from build123d import *

# Parameters (mm, degrees)
F0_R     = 20
F0_R_2   = 3
F1_DEPTH = 15
F2_R     = 1.5
F3_DEPTH = 15
F4_COUNT = 30


with BuildPart() as f1:
    # F0 (on Front) → F1 (new body)
    with BuildSketch(Plane.XZ):
        Circle(F0_R)
        Circle(F0_R_2, mode=Mode.SUBTRACT)
    extrude(amount=F1_DEPTH)


with BuildPart() as f3:
    # F2 (on face) → F3 (new body, through all)
    with BuildSketch(Plane.XZ.offset(15)):
        with Locations((20.171481, 1.781533)):
            Circle(F2_R)
    extrude(amount=-F3_DEPTH)


with BuildPart() as f4_1:
    # F4: instance of F3
    add(f3.part.rotate(Axis((0, 0, 0), (0, 1, 0)), 1 * 360 / F4_COUNT))


with BuildPart() as f4_2:
    # F4: instance of F3
    add(f3.part.rotate(Axis((0, 0, 0), (0, 1, 0)), 2 * 360 / F4_COUNT))


with BuildPart() as f4_3:
    # F4: instance of F3
    add(f3.part.rotate(Axis((0, 0, 0), (0, 1, 0)), 3 * 360 / F4_COUNT))


with BuildPart() as f4_4:
    # F4: instance of F3
    add(f3.part.rotate(Axis((0, 0, 0), (0, 1, 0)), 4 * 360 / F4_COUNT))


with BuildPart() as f4_5:
    # F4: instance of F3
    add(f3.part.rotate(Axis((0, 0, 0), (0, 1, 0)), 5 * 360 / F4_COUNT))


with BuildPart() as f4_6:
    # F4: instance of F3
    add(f3.part.rotate(Axis((0, 0, 0), (0, 1, 0)), 6 * 360 / F4_COUNT))


with BuildPart() as f4_7:
    # F4: instance of F3
    add(f3.part.rotate(Axis((0, 0, 0), (0, 1, 0)), 7 * 360 / F4_COUNT))


with BuildPart() as f4_8:
    # F4: instance of F3
    add(f3.part.rotate(Axis((0, 0, 0), (0, 1, 0)), 8 * 360 / F4_COUNT))


with BuildPart() as f4_9:
    # F4: instance of F3
    add(f3.part.rotate(Axis((0, 0, 0), (0, 1, 0)), 9 * 360 / F4_COUNT))


with BuildPart() as f4_10:
    # F4: instance of F3
    add(f3.part.rotate(Axis((0, 0, 0), (0, 1, 0)), 10 * 360 / F4_COUNT))


with BuildPart() as f4_11:
    # F4: instance of F3
    add(f3.part.rotate(Axis((0, 0, 0), (0, 1, 0)), 11 * 360 / F4_COUNT))


with BuildPart() as f4_12:
    # F4: instance of F3
    add(f3.part.rotate(Axis((0, 0, 0), (0, 1, 0)), 12 * 360 / F4_COUNT))


with BuildPart() as f4_13:
    # F4: instance of F3
    add(f3.part.rotate(Axis((0, 0, 0), (0, 1, 0)), 13 * 360 / F4_COUNT))


with BuildPart() as f4_14:
    # F4: instance of F3
    add(f3.part.rotate(Axis((0, 0, 0), (0, 1, 0)), 14 * 360 / F4_COUNT))


with BuildPart() as f4_15:
    # F4: instance of F3
    add(f3.part.rotate(Axis((0, 0, 0), (0, 1, 0)), 15 * 360 / F4_COUNT))


with BuildPart() as f4_16:
    # F4: instance of F3
    add(f3.part.rotate(Axis((0, 0, 0), (0, 1, 0)), 16 * 360 / F4_COUNT))


with BuildPart() as f4_17:
    # F4: instance of F3
    add(f3.part.rotate(Axis((0, 0, 0), (0, 1, 0)), 17 * 360 / F4_COUNT))


with BuildPart() as f4_18:
    # F4: instance of F3
    add(f3.part.rotate(Axis((0, 0, 0), (0, 1, 0)), 18 * 360 / F4_COUNT))


with BuildPart() as f4_19:
    # F4: instance of F3
    add(f3.part.rotate(Axis((0, 0, 0), (0, 1, 0)), 19 * 360 / F4_COUNT))


with BuildPart() as f4_20:
    # F4: instance of F3
    add(f3.part.rotate(Axis((0, 0, 0), (0, 1, 0)), 20 * 360 / F4_COUNT))


with BuildPart() as f4_21:
    # F4: instance of F3
    add(f3.part.rotate(Axis((0, 0, 0), (0, 1, 0)), 21 * 360 / F4_COUNT))


with BuildPart() as f4_22:
    # F4: instance of F3
    add(f3.part.rotate(Axis((0, 0, 0), (0, 1, 0)), 22 * 360 / F4_COUNT))


with BuildPart() as f4_23:
    # F4: instance of F3
    add(f3.part.rotate(Axis((0, 0, 0), (0, 1, 0)), 23 * 360 / F4_COUNT))


with BuildPart() as f4_24:
    # F4: instance of F3
    add(f3.part.rotate(Axis((0, 0, 0), (0, 1, 0)), 24 * 360 / F4_COUNT))


with BuildPart() as f4_25:
    # F4: instance of F3
    add(f3.part.rotate(Axis((0, 0, 0), (0, 1, 0)), 25 * 360 / F4_COUNT))


with BuildPart() as f4_26:
    # F4: instance of F3
    add(f3.part.rotate(Axis((0, 0, 0), (0, 1, 0)), 26 * 360 / F4_COUNT))


with BuildPart() as f4_27:
    # F4: instance of F3
    add(f3.part.rotate(Axis((0, 0, 0), (0, 1, 0)), 27 * 360 / F4_COUNT))


with BuildPart() as f4_28:
    # F4: instance of F3
    add(f3.part.rotate(Axis((0, 0, 0), (0, 1, 0)), 28 * 360 / F4_COUNT))


with BuildPart() as f4_29:
    # F4: instance of F3
    add(f3.part.rotate(Axis((0, 0, 0), (0, 1, 0)), 29 * 360 / F4_COUNT))


with BuildPart() as f1_1:
    add(f1.part)

    # F5: cut F4_15, F4_16, F4_17, F4_18, F4_19, F4_20, F4_21, F4_23, F4_25, F4_22, F4_24, F4_26, F4_27, F4_28, F4_29, F3, F4_1, F4_2, F4_3, F4_4, F4_5, F4_6, F4_7, F4_8, F4_9, F4_10, F4_11, F4_12, F4_13, F4_14
    add(f4_15.part, mode=Mode.SUBTRACT)
    add(f4_16.part, mode=Mode.SUBTRACT)
    add(f4_17.part, mode=Mode.SUBTRACT)
    add(f4_18.part, mode=Mode.SUBTRACT)
    add(f4_19.part, mode=Mode.SUBTRACT)
    add(f4_20.part, mode=Mode.SUBTRACT)
    add(f4_21.part, mode=Mode.SUBTRACT)
    add(f4_23.part, mode=Mode.SUBTRACT)
    add(f4_25.part, mode=Mode.SUBTRACT)
    add(f4_22.part, mode=Mode.SUBTRACT)
    add(f4_24.part, mode=Mode.SUBTRACT)
    add(f4_26.part, mode=Mode.SUBTRACT)
    add(f4_27.part, mode=Mode.SUBTRACT)
    add(f4_28.part, mode=Mode.SUBTRACT)
    add(f4_29.part, mode=Mode.SUBTRACT)
    add(f3.part, mode=Mode.SUBTRACT)
    add(f4_1.part, mode=Mode.SUBTRACT)
    add(f4_2.part, mode=Mode.SUBTRACT)
    add(f4_3.part, mode=Mode.SUBTRACT)
    add(f4_4.part, mode=Mode.SUBTRACT)
    add(f4_5.part, mode=Mode.SUBTRACT)
    add(f4_6.part, mode=Mode.SUBTRACT)
    add(f4_7.part, mode=Mode.SUBTRACT)
    add(f4_8.part, mode=Mode.SUBTRACT)
    add(f4_9.part, mode=Mode.SUBTRACT)
    add(f4_10.part, mode=Mode.SUBTRACT)
    add(f4_11.part, mode=Mode.SUBTRACT)
    add(f4_12.part, mode=Mode.SUBTRACT)
    add(f4_13.part, mode=Mode.SUBTRACT)
    add(f4_14.part, mode=Mode.SUBTRACT)

    # F6 (on Right) → F7 (revolve)
    with BuildSketch(Plane.YZ):
        Polygon((-15, 3), (-15, 0), (90, 0), (90, 16), (40, 16), (40, 15), (10, 15), (10, 3), align=None)
    revolve(axis=Axis((0, 37.5, 0), (0, 1, 0)))


solid = f1_1.part
Part model, mm, in its own coordinate system. A direction names the side the tool comes from. Coordinates: 2 decimals unless noted, no trailing zeros. Order: outer loops, then holes, each group sorted by start corner. A loop starts at its lowest first (then second) coordinate and runs counter-clockwise, first axis right, second up. Notation, with made-up numbers: M -17,13.5 L -10,13.5 A24 cw -10,29.5 Z; hole C 13,-38 d5. An arc over 180 degrees is marked long. Use a Markdown table: item, result.
(1) Probe L1, parallel to Y at x = 11, z = -4; L2, parallel to Y at x = 18.5, z = -4; L3, parallel to X at y = 2, z = 0. List the from-to ranges inside material, lowest first.
A:
| item | result |
|---|---|
| L1 | y = -15 to 0, 10 to 90 |
| L2 | y = -15 to 0 |
| L3 | x = -3 to 3 |
(2) Cut at B-B on y = 3. Write the cut outline in (x, z).
A:
| item | result |
|---|---|
| outline | C 0,0 d6 |
(3) Tool access for faces 1 (the cylindrical face through (-10.791, -7.605, 15.334)), 2 (the cylindrical face through (0.9, 4.93, 2.86)): list every direction of +Z, -Z, +X, -X, +Y, -Y with a clear straight run to the whole face (end or side of a thin tool).
A:
| item | result |
|---|---|
| face 1 | +Y, -Y |
| face 2 | none |
(4) Pull direction Z, two halves, no side cores. Call faces 3 (the flat face through (0, -15, 0)), 4 (the cylindrical face through (13.7, -7.6, -12.8)), 5 (the cylindrical face through (3.6, -7.6, -18.4)), 6 (the cylindrical face through (16.378, -7.605, 9.129)): released by +Z, released by -Z, zero draft, split by the parting line, or undercut.
A:
| item | result |
|---|---|
| face 3 | zero draft |
| face 4 | undercut |
| face 5 | released by -Z |
| face 6 | undercut |
(5) Cut at A-A on x = 0. Write the cut outline in (y, z), then the cut area to 3 significant figures.
A:
| item | result |
|---|---|
| outline | M -15,-18.79 L 0,-18.79 L 0,-3 L 10,-3 L 10,-15 L 40,-15 L 40,-16 L 90,-16 L 90,16 L 40,16 L 40,15 L 10,15 L 10,3 L 0,3 L 0,18.79 L -15,18.79 Z |
| area | 3,120 mm^2 |
(6) Cut at C-C on y = 35.5. Write the cut outline in (x, z).
A:
| item | result |
|---|---|
| outline | C 0,0 d30 |
(7) Flat gauge pins, fed straight in: pin 1 (12 mm diameter, centred on x = -15, z = 15, fed in from +Y); pin 2 (5 mm diameter, centred on x = 3.5, y = 56.5, fed in from +Z); pin 3 (1 mm diameter, centred on y = 46, z = -2.5, fed in from +X); pin 4 (2 mm diameter, centred on x = 6, y = -1.5, fed in from +Z). Where does each tip first touch, or does it go through?
A:
| item | result |
|---|---|
| pin 1 | stops at y = 90 |
| pin 2 | stops at z = 15.97 |
| pin 3 | stops at x = 15.87 |
| pin 4 | stops at z = 19.11 |
